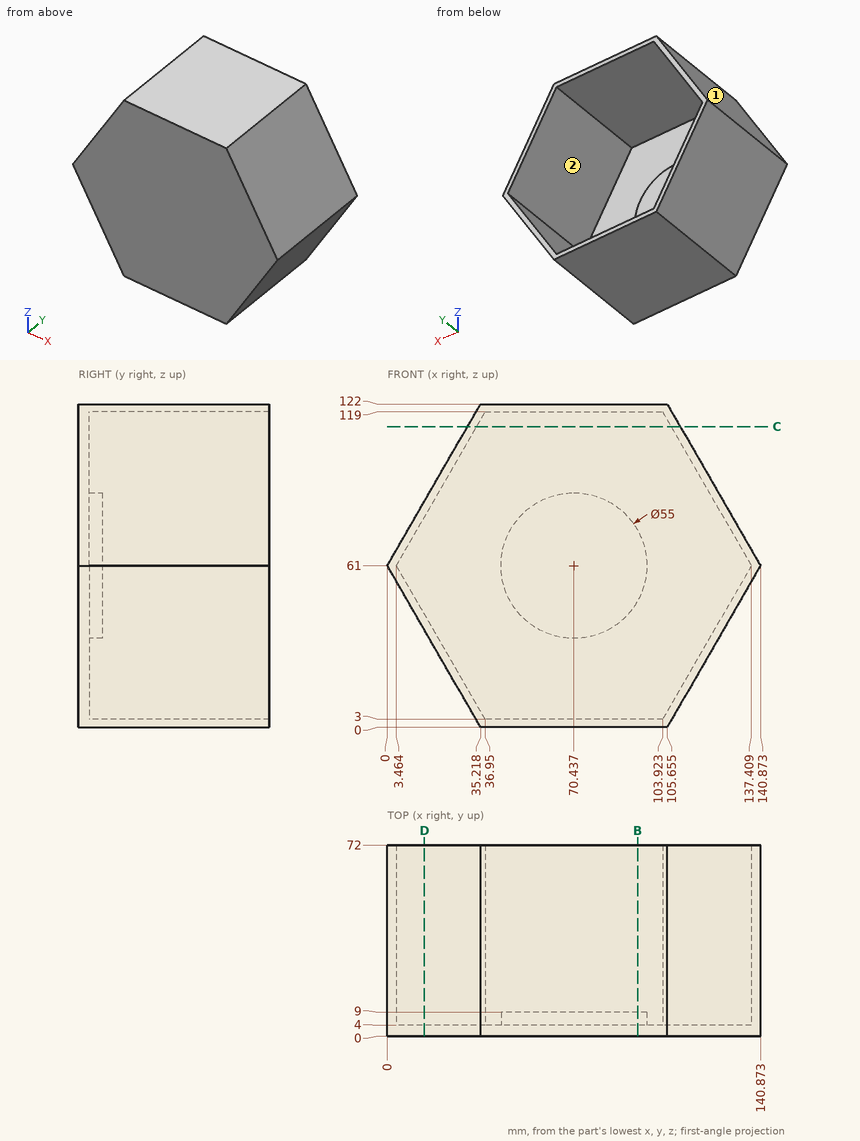
Source: three-view drawing plus pictorial views. Frame: mm from the lowest corner of the part. A direction names the side the tool comes from. Give positions to 0.01 mm unless a question says otherwise; leave off trailing zeros. Loops run counter-clockwise (first coordinate to the right, second up) from the corner with the lowest first, then second, coordinate; pieces in that order, holes last. Notation, with made-up numbers: M 8.5,66.25 L 43.5,66.25 A34 ccw 43.5,96.25 Z; hole C -4.5,54 d1. An arc over 180 degrees is marked long. Put each result on its own line as item: value.
Q1. Section D-D (x = 14). Return the cut outline in (y, z), and give its area (3 significant figures).
Response values:
outline: M 0,36.75 L 72,36.75 L 72,42.75 L 4,42.75 L 4,79.25 L 72,79.25 L 72,85.25 L 0,85.25 Z
area: 1,010 mm²
Q2. Reachability of the marked faces 1 and 2 from +Z, -Z, +X, -X, +Y, -Y: full face, straight path, thin tool, end or side. Return the list, or none.
Response values:
face 1: +Z, -X, +Y, -Y
face 2: +Y
Q3. Pin query (flat end, axial travel): P1, Ø4, axis at y = 56.5, z = 80, coming from the +X side; P2, Ø6, axis at x = 30.5, y = 44.5, coming from the +Z side (1 decimal); P3, Ø8, axis at y = 20, z = 24.5, coming from the +X side. Return the tip coordinate at first contact, or that it passes through.
Response values:
P1: stops at x = 131.06
P2: stops at z = 119
P3: stops at x = 122.11
Q4. Line query: probe 1 along Z at (x, y) = (56, 26.5); probe 2 along Z at (x, y) = (89.5, 4.5); probe 3 along Y at (x, z) = (92.5, 99.5). Output: solid intervals per line, ascending. Write a range as [from, to].
Response values:
probe 1: z = [0, 3], [119, 122]
probe 2: z = [0, 3], [41.18, 80.82], [119, 122]
probe 3: y = [0, 4]
Q5. Section C-C (z = 113.5). Return the cut outline in (x, y) (1 decimal).
Response values:
outline: M 30.3,0 L 110.6,0 L 110.6,72 L 107.1,72 L 107.1,4 L 33.8,4 L 33.8,72 L 30.3,72 Z
Q6. Section B-B (x = 94.5). Return the cut outline in (y, z), and give its area (3 significant figures).
Response values:
outline: M 0,0 L 72,0 L 72,3 L 4,3 L 4,47.69 L 9,47.69 L 9,74.31 L 4,74.31 L 4,119 L 72,119 L 72,122 L 0,122 Z
area: 1,030 mm²
